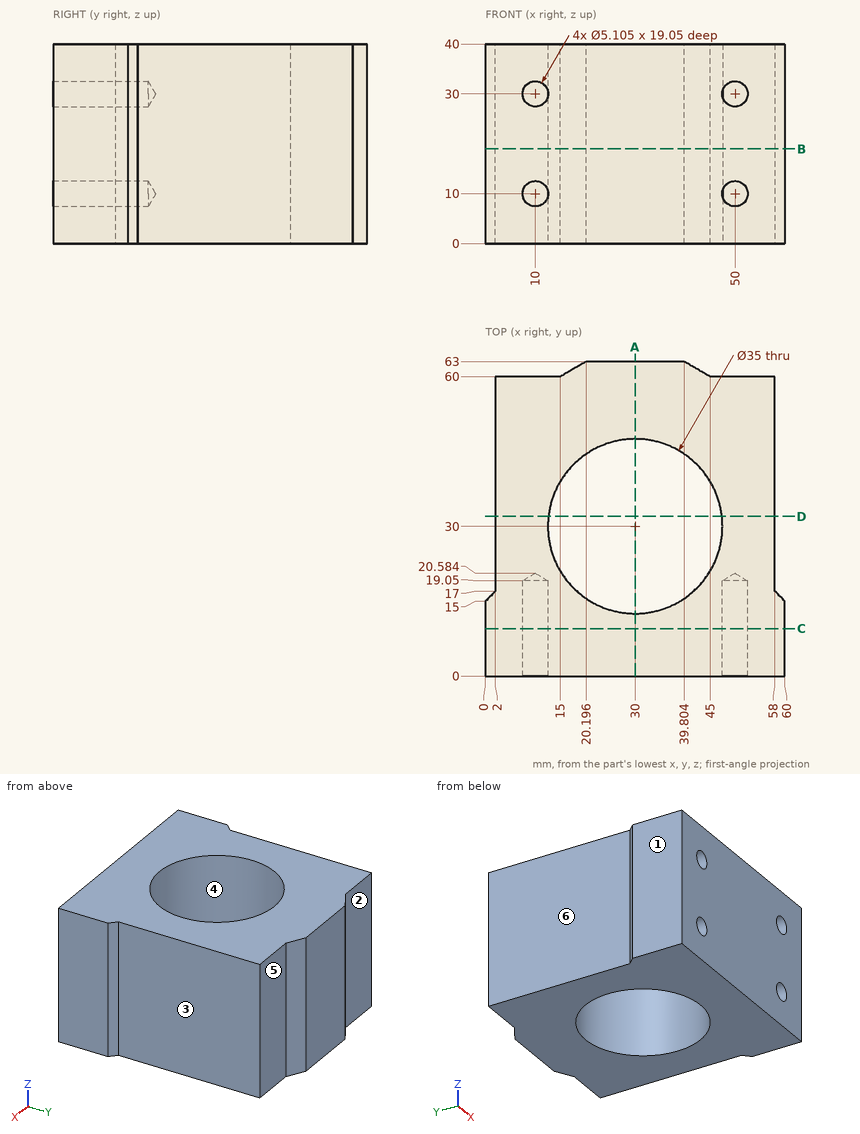
Print and shaded views of the part. All mm, measured from the part's lowest x, y and z. A direction names the side the tool comes from. Round coordinates to 2 decimals unless told otherwise and drop trailing zeros. Write each loop counter-clockwise with the first axis right and the second up, starting at its lowest first coordinate (ties: lowest second). Pieces come first, ordered by that corner, then holes. Notation, with made-up numbers: (-9, 38) - (40, 38) arc R7 cw to (40, 50) - close; hole circle Ø6 at (-3, 65.5). An arc over 180 degrees is marked (long way). Use CSV: the item, a comma, the result in double quotes. Start each with the question number.
Item 1: Two-plate mould, pull along X, no slides. Class the marked faces 3, 4, 5 and 6: released by +X, released by -X, zero draft, split by the parting line, or undercut.
Item 2: Band-saw the part on A-A (x = 30). Write the cut outline in (y, z).
Item 3: Pin check, flat tips, straight feed: P1, Ø12, axis at y = 28, z = 8, coming from the -X side; P2, Ø6.5, axis at x = 6.5, z = 23.5, coming from the +Y side; P3, Ø4, axis at x = 50, z = 10, coming from the -Y side. Stop position of each tip, or through.
Item 4: Band-saw the part on C-C (y = 9.5). Write the cut outline in (x, z) (1 decimal), and give its area (3 significant figures).
Item 5: Band-saw the part on D-D (y = 32). Write the cut outline in (x, z) (1 decimal), and give its area (3 significant figures).
Item 6: Drill centre lines: L1, parallel to X at y = 7.75, z = 10; L2, parallel to Z at x = 10, y = 7.25; L3, parallel to Y at x = 39, z = 27. Where is each one in solid material? Low to high. Write a range as [from, to].
Item 7: Band-saw the part on B-B (z = 19). Write the cut outline in (x, y), and give its area (3 significant figures).
Item 8: Tool access for the marked faces 1 and 2: list every direction of +Z, -Z, +X, -X, +Y, -Y with a clear straight run to the whole face (end or side of a thin tool).
Checked values:
1,face 3,"released by +X"
1,face 4,"undercut"
1,face 5,"zero draft"
1,face 6,"released by -X"
2,outline,"(0, 0) - (12.5, 0) - (12.5, 40) - (0, 40) - close; (47.5, 0) - (63, 0) - (63, 40) - (47.5, 40) - close"
3,P1,"stops at x = 2"
3,P2,"stops at y = 60"
3,P3,"stops at y = 19.38"
4,outline,"(0, 0) - (60, 0) - (60, 40) - (0, 40) - close; hole circle Ø5.1 at (10, 10); hole circle Ø5.1 at (10, 30); hole circle Ø5.1 at (50, 10); hole circle Ø5.1 at (50, 30)"
4,area,"2,320 mm²"
5,outline,"(2, 0) - (12.6, 0) - (12.6, 40) - (2, 40) - close; (47.4, 0) - (58, 0) - (58, 40) - (47.4, 40) - close"
5,area,"849 mm²"
6,L1,"x = [0, 7.45], [12.55, 47.45], [52.55, 60]"
6,L2,"z = [0, 7.45], [12.55, 27.45], [32.55, 40]"
6,L3,"y = [0, 14.99], [45.01, 63]"
7,outline,"(0, 0) - (60, 0) - (60, 15) - (58, 17) - (58, 60) - (45, 60) - (39.8, 63) - (20.2, 63) - (15, 60) - (2, 60) - (2, 17) - (0, 15) - close; hole circle Ø35 at (30, 30)"
7,area,"2,540 mm²"
8,face 1,"+Z, -Z, -X, +Y, -Y"
8,face 2,"+Z, -Z, -X, +Y"
